from build123d import *

# Parameters (mm, degrees)
SKIZZE1_W                       = 65
SKIZZE1_H                       = 15
AUFSATZ_LINEAR_AUSTRAGEN1_DEPTH = 4
SCHNITT_LINEAR_AUSTRAGEN1_REACH = 6
SKIZZE2_W                       = 7.5
SKIZZE2_H                       = 5


with BuildPart() as part:
    # Skizze1 → Aufsatz-Linear austragen1 (new body)
    with BuildSketch(Plane.XY):
        with Locations((32.5, 7.5)):
            Rectangle(SKIZZE1_W, SKIZZE1_H)
    extrude(amount=AUFSATZ_LINEAR_AUSTRAGEN1_DEPTH)

    # Skizze2 → Schnitt-Linear austragen1 (cut, up to next)
    with BuildSketch(Plane.XY.offset(4), mode=Mode.PRIVATE) as schnitt_linear_austragen1_sk1:
        with Locations((32.5, 12.5)):
            Rectangle(SKIZZE2_W, SKIZZE2_H)
    schnitt_linear_austragen1_tool1 = extrude(schnitt_linear_austragen1_sk1.sketch, amount=-SCHNITT_LINEAR_AUSTRAGEN1_REACH, mode=Mode.PRIVATE) & part.part
    add(schnitt_linear_austragen1_tool1.solids().sort_by_distance((32.5, 12.5, 4))[0], mode=Mode.SUBTRACT)


solid = part.part
Check sheet for the modelled part. Datum: model origin and axes. Units: mm. A direction names the side the tool comes from. Round coordinates to 2 decimals unless told otherwise and drop trailing zeros. Loops run counter-clockwise (first coordinate to the right, second up) from the corner with the lowest first, then second, coordinate; pieces in that order, holes last. Notation, with made-up numbers: (63.25, -38.5) - (102.25, -38.5) arc R11 cw to (102.25, -24.5) - close; hole circle Ø9 at (70, -20.5). An arc over 180 degrees is marked (long way). Answer as CSV lines item,"result". Start each with the question number.
Item 1: Release check for a two-part mould opening along X. For faces 3 (the flat face through (32, 8, 0)), 4 (the flat face through (28.75, 12, 2)), 5 (the flat face through (0, 7, 2)) record: +X half, -X half, draft (parallel to the pull), parting line (faces both ways), or undercut.
Item 2: Set-up check for faces 1 (the flat face through (36.25, 12, 2)), 2 (the flat face through (32, 8, 4)): record each of +Z, -Z, +X, -X, +Y, -Y from which the full face is reachable in a straight line by a thin tool's end or side.
Item 3: Section check B-B (z = 1.2). Record the boundary of the cut face in (x, y), and give its area (4 significant figures).
Item 4: Scan line: line 1 (X direction, y = 14, z = 3.1). Record every from-to range of solid material in increasing order. Write a range as [from, to].
Item 5: Section check A-A (y = 13.25). Record the boundary of the cut face in (x, z), and give its area (3 significant figures).
Report:
1,face 3,"draft"
1,face 4,"undercut"
1,face 5,"-X half"
2,face 1,"+Z, -Z, +Y"
2,face 2,"+Z, +X, -X, +Y, -Y"
3,outline,"(0, 0) - (65, 0) - (65, 15) - (36.25, 15) - (36.25, 10) - (28.75, 10) - (28.75, 15) - (0, 15) - close"
3,area,"937.5 mm2"
4,line 1,"x = [0, 28.75], [36.25, 65]"
5,outline,"(0, 0) - (28.75, 0) - (28.75, 4) - (0, 4) - close; (36.25, 0) - (65, 0) - (65, 4) - (36.25, 4) - close"
5,area,"230 mm2"
